The model under review builds one solid part; all positions refer to its coordinate system, in mm. A direction names the side the tool comes from. Round coordinates to 2 decimals unless told otherwise and drop trailing zeros. Write each loop counter-clockwise with the first axis right and the second up, starting at its lowest first coordinate (ties: lowest second). Pieces come first, ordered by that corner, then holes.
Item 1: Add section C-C (x = -48). Give the boundary of the cut face in (y, z), plus the area to 4 significant figures.
Item 2: Draft analysis for pull direction X (two halves, no side actions). For faces 5 (the face through (-115, 108, 12)), 6 (the face through (-126.268, 69.795, 43.908)), 7 (the face through (127, 5, 27)), state which applies: +X half, -X half, draft (parallel to the pull), parting line (faces both ways), or undercut.
Item 3: Clearance check with flat-ended pins moving along their axes: pin 1 Ø2 at (x, y) = (59.5, -54) entering from +Z; pin 2 Ø3.5 at (x, y) = (121.5, 110) entering from +Z; pin 3 Ø16.5 at (x, z) = (51, 33) entering from +Y. State where each tip first meets the part, or that it passes through.
Item 4: To check wall thickness, follow L1, parallel to X at y = -33.5, z = 8.5; L2, parallel to X at y = -66, z = 23; L3, parallel to Z at x = -2, y = 96.5. State the ranges of each line that lie inside material, in increasing order.
Item 5: Machinability: for faces 1 (the face through (-2, 2, -2.5)), 2 (the face through (-107.815, 109.521, 19.189)), 3 (the face through (115, 108, 12)), 4 (the face through (-127, 5, 27)), which of the approach directions +Z, -Z, +X, -X, +Y, -Y give a long, thin tool a straight path to every point of the face, cutting with its end or side? Answer none if there is none.
Item 6: Add section B-B (z = 51). Give the boundary of the cut face in (x, y), plus the area to 3 significant figures.
```python
from build123d import *

# Parameters (mm, degrees)
SKETCH1_W                               = 255
SKETCH1_H                               = 222
BOSS_EXTRUDE1_DEPTH                     = 2.5
SKETCH2_W                               = 2.5
SKETCH2_H                               = 222
SKETCH2_W_2                             = 250
SKETCH2_H_2                             = 2.5
BOSS_EXTRUDE2_DEPTH                     = 55
HOLD_TAB_DEPTH                          = 3
FRONT_TAPER_DEPTH                       = 178.770216853
FRONT_TAPER_DEPTH_BACK                  = 178.770216853
SKETCH6_W                               = 8.4
SKETCH6_H                               = 204.4
MOUNTING_POCKET_DEPTH                   = 284.048140782
PRINT_CHAMFERS_SIZE                     = 0.5
PRINT_CHAMFERS_OF_MOUNTING_POCKETS_SIZE = 0.5


with BuildPart() as part:
    # Sketch1 → Boss-Extrude1 (new body)
    with BuildSketch(Plane.XY):
        Rectangle(SKETCH1_W, SKETCH1_H)
    extrude(amount=-BOSS_EXTRUDE1_DEPTH)

    # Sketch2 → Boss-Extrude2 (add)
    with BuildSketch(Plane.XY):
        with Locations((-126.25, 0)):
            Rectangle(SKETCH2_W, SKETCH2_H)
        with Locations((0, -109.75)):
            Rectangle(SKETCH2_W_2, SKETCH2_H_2)
        with Locations((126.25, 0)):
            Rectangle(SKETCH2_W, SKETCH2_H)
    extrude(amount=BOSS_EXTRUDE2_DEPTH)

    # Sketch4 → Hold Tab (add)
    with BuildSketch(Plane(origin=(0, 111, 0), x_dir=(1, 0, 0), z_dir=(0, 1, 0))):
        Polygon((127.5, 2.5), (127.5, -32.5), (115.5, -32.5), (99.911542732, -5.5), (99.911542732, 2.5), align=None)
    hold_tab = extrude(amount=-HOLD_TAB_DEPTH)

    # Hold Tabs: Hold Tab across plane
    add(hold_tab.mirror(Plane(origin=(0, 0, 0), x_dir=(0, 0, 1), z_dir=(1, 0, 0))))

    # Sketch5 → Front Taper (cut, two sides: drawn at the far end of the back side and taken through both)
    with BuildSketch(Plane(origin=(0, 0, 0), x_dir=(0, 0, -1), z_dir=(1, 0, 0)).offset(-FRONT_TAPER_DEPTH_BACK)):
        Polygon((-55, 29.727996643), (-32.5, 111), (-55, 111), align=None)
    extrude(amount=FRONT_TAPER_DEPTH + FRONT_TAPER_DEPTH_BACK, mode=Mode.SUBTRACT)

    # Sketch6 → Mounting Pocket (cut, through all)
    with BuildSketch(Plane.ZY.offset(-127)):
        with Locations((27, 4)):
            Rectangle(SKETCH6_W, SKETCH6_H)
    mounting_pocket = extrude(amount=-MOUNTING_POCKET_DEPTH, mode=Mode.SUBTRACT)

    # Print Chamfers
    print_chamfers_edges = [part.edges().sort_by_distance(p)[0] for p in [
        (127.5, 106.2, 27),
        (127.5, 4, 22.8),
        (127.5, -98.2, 27),
        (127.5, 4, 31.2),
    ]]
    chamfer(print_chamfers_edges, length=PRINT_CHAMFERS_SIZE - 0.0001)  # a hair under: the kernel refuses the full size

    # Mounting Pockets: Mounting Pocket across plane
    add(mounting_pocket.mirror(Plane(origin=(0, 0, 0), x_dir=(0, 0, 1), z_dir=(1, 0, 0))), mode=Mode.SUBTRACT)

    # Print Chamfers of Mounting Pockets
    print_chamfers_of_mounting_pockets_edges = [part.edges().sort_by_distance(p)[0] for p in [
        (-127.5, 106.2, 27),
        (-127.5, 4, 22.8),
        (-127.5, -98.2, 27),
        (-127.5, 4, 31.2),
    ]]
    chamfer(print_chamfers_of_mounting_pockets_edges, length=PRINT_CHAMFERS_OF_MOUNTING_POCKETS_SIZE - 0.0001)  # a hair under: the kernel refuses the full size


solid = part.part
```
Numbers:
1. outline: (-111, -2.5) - (111, -2.5) - (111, 0) - (-108.5, 0) - (-108.5, 55) - (-111, 55) - close
1. area: 692.5 mm2
2. face 5: undercut
2. face 6: draft
2. face 7: +X half
3. pin 1: stops at z = 0
3. pin 2: stops at z = 32.5
3. pin 3: stops at y = -108.5
4. L1: x = -127.5 to -125, 125 to 127.5
4. L2: x = -127 to -125, 125 to 127
4. L3: z = -2.5 to 0
5. face 1: -Z, +X, -X, +Y, -Y
5. face 2: +Z, +Y
5. face 3: +Z
5. face 4: -X
6. outline: (-127.5, -111) - (127.5, -111) - (127.5, 44.18) - (125, 44.18) - (125, -108.5) - (-125, -108.5) - (-125, 44.18) - (-127.5, 44.18) - close
6. area: 1,400 mm2
